Could you check a few things on this drawing? It's one solid part, dimensions in mm from its lowest x, y, z. Round coordinates to 2 decimals unless told otherwise and drop trailing zeros. Loops run counter-clockwise (first coordinate to the right, second up) from the corner with the lowest first, then second, coordinate; pieces in that order, holes last. Notation, with made-up numbers: M 21.5,54.25 L 38.5,54.25 A29 cw 38.5,88.25 Z; hole C -25,70 d2. An arc over 180 degrees is marked long. Use a Markdown table: item, result. Add a question column.
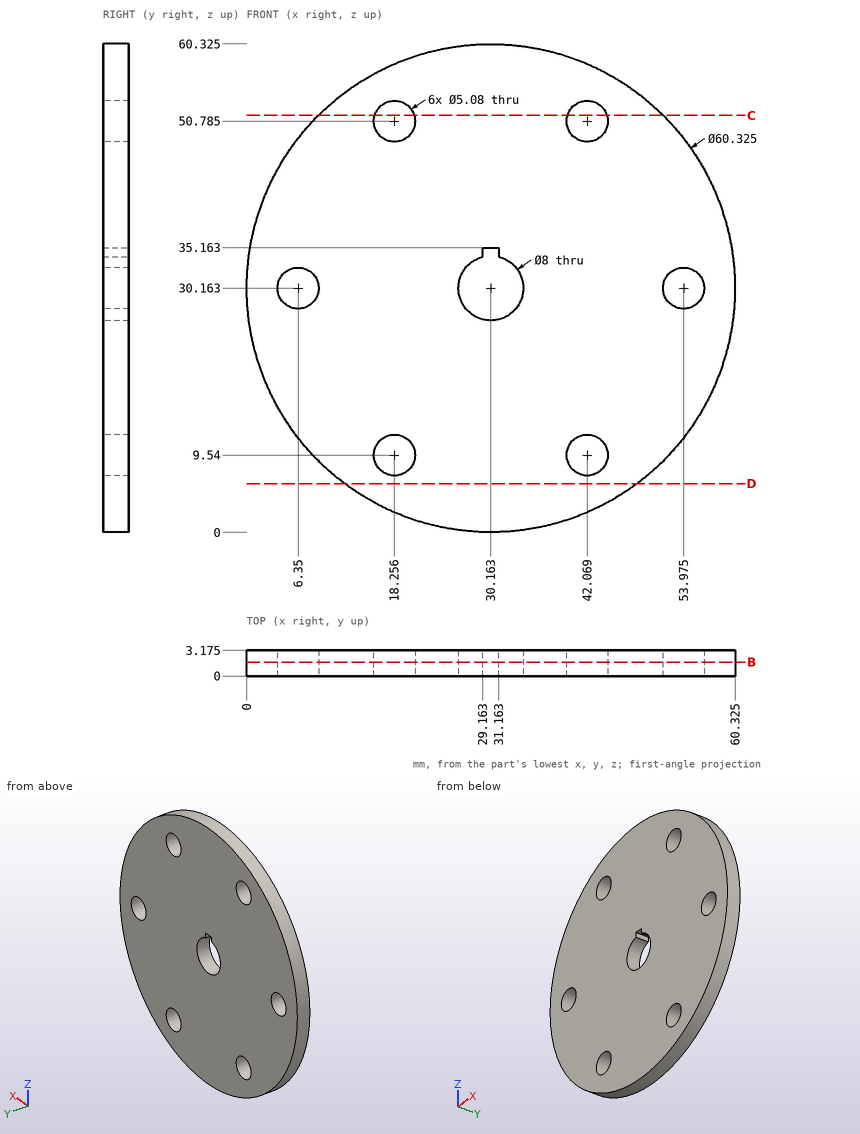
(1) If I drill on probe 1 along X at (y, z) = (2, 30) (1 decimal); probe 2 along Z at (x, y) = (30.5, 0.3); probe 3 along X at (y, z) = (0.8, 10) (1 decimal), over which ranges is the centre line in solid material (lowest first)? Write a range as [from, to].
(2) I'm going to push flat-ended pins straight in: pin 1 (0.6 mm diameter, centred on x = 30.5, y = 2, fed in from -Z); pin 2 (0.9 mm diameter, centred on y = 2, z = 34.5, fed in from -X); pin 3 (1.2 mm diameter, centred on y = 1, z = 35, fed in from +X). Where does each tip first touch, or does it pass through?
(3) Suppose I cut it at C-C on z = 51.5. List the corners of the cut face in (x, y) for me (1 decimal).
(4) Suppose I cut it at B-B on y = 1.7. Count the separate pieces of the cut face and the enclosed holes in it, and give its area (3 significant figures).
(5) Suppose I cut it at D-D on z = 6. List the corners of the cut face in (x, y) for me (1 decimal).
Results below:
| question | item | result |
|---|---|---|
| 1 | probe 1 | x = [0, 3.8], [8.9, 26.2], [34.2, 51.4], [56.5, 60.3] |
| 1 | probe 2 | z = [0, 26.18], [35.16, 60.32] |
| 1 | probe 3 | x = [7.7, 15.8], [20.8, 39.6], [44.6, 52.6] |
| 2 | pin 1 | stops at z = 0 |
| 2 | pin 2 | stops at x = 0.25 |
| 2 | pin 3 | stops at x = 60.03 |
| 3 | outline | M 8.8,0 L 15.8,0 L 15.8,3.2 L 8.8,3.2 Z; M 20.7,0 L 39.6,0 L 39.6,3.2 L 20.7,3.2 Z; M 44.5,0 L 51.5,0 L 51.5,3.2 L 44.5,3.2 Z |
| 4 | separate pieces | 1 |
| 4 | enclosed holes | 7 |
| 4 | area | 2,680 mm² |
| 5 | outline | M 12.1,0 L 48.2,0 L 48.2,3.2 L 12.1,3.2 Z |
